Could you check a few things on this model? Use its own coordinates, in mm. Give positions to 0.01 mm unless a question says otherwise; leave off trailing zeros. Order: outer loops, then holes, each group sorted by start corner. A loop starts at its lowest first (then second) coordinate and runs counter-clockwise, first axis right, second up. Notation, with made-up numbers: M 11,21.5 L 43,21.5 A26 ccw 43,57.5 Z; hole C 54,28.5 d5. An arc over 180 degrees is marked long. Use a Markdown table: item, result. Add a question column.
```python
from build123d import *

# Parameters (mm, degrees)
SKETCH1_R           = 2.5
BOSS_EXTRUDE1_DEPTH = 4


with BuildPart() as part:
    # Sketch1 → Boss-Extrude1 (new body)
    with BuildSketch(Plane(origin=(0, 0, 0), x_dir=(1, 0, 0), z_dir=(0, 1, 0))):
        Polygon((-370, -69), (-370, -30), (-328, -30), (-328, 70), (370, 70), (370, -69), (349, -69), (349, -90), (-110, -90), (-110, -69), (-131, -69), (-131, -90), (-349, -90), (-349, -69), align=None)
        with Locations((-340, -80)):
            Circle(SKETCH1_R, mode=Mode.SUBTRACT)
        with Locations((0, -80)):
            Circle(SKETCH1_R, mode=Mode.SUBTRACT)
        with Locations((340, -80)):
            Circle(SKETCH1_R, mode=Mode.SUBTRACT)
    extrude(amount=BOSS_EXTRUDE1_DEPTH)


solid = part.part
```
1) Please list where these lines run through material, in increasing order: line 1 (X direction, y = 3.1, z = 80); line 2 (Z direction, x = -340, y = 1.7); line 3 (Z direction, x = 0, y = 2.45). Write a range as from..to.
2) Suppose I cut it at B-B on z = -14. Please give me the cut outline in (x, y).
3) For pin 1 (2 mm diameter, centred on y = 2, z = 84, fed in from -X); pin 2 (3 mm diameter, centred on x = 0, z = 80, fed in from -Y); pin 3 (2 mm diameter, centred on y = 1, z = 3, fed in from -X); pin 4 (1.2 mm diameter, centred on x = -119.5, y = 1.5, fed in from +Z), each with a flat end and sliding along its axis, tell me the tip position at first contact or that it passes through.
4) Suppose I cut it at A-A on y = 2.1. Please give me the cut outline in (x, z).
Values found:
| question | item | result |
|---|---|---|
| 1 | line 1 | x = -349..-342.5, -337.5..-131, -110..-2.5, 2.5..337.5, 342.5..349 |
| 1 | line 2 | z = 30..77.5, 82.5..90 |
| 1 | line 3 | z = -70..77.5, 82.5..90 |
| 2 | outline | M -328,0 L 370,0 L 370,4 L -328,4 Z |
| 3 | pin 1 | stops at x = -349 |
| 3 | pin 2 | passes through |
| 3 | pin 3 | stops at x = -328 |
| 3 | pin 4 | stops at z = 69 |
| 4 | outline | M -370,30 L -328,30 L -328,-70 L 370,-70 L 370,69 L 349,69 L 349,90 L -110,90 L -110,69 L -131,69 L -131,90 L -349,90 L -349,69 L -370,69 Z; hole C -340,80 d5; hole C 0,80 d5; hole C 340,80 d5 |
